from build123d import *

# Parameters (mm, degrees)
SKETCH1_W           = 15
SKETCH1_H           = 15
BOSS_EXTRUDE1_DEPTH = 2
FILLET11_R          = 5
FILLET13_R          = 2
SKETCH7_W           = 8.5
SKETCH7_H           = 7.5
BOSS_EXTRUDE5_DEPTH = 5
CUT_EXTRUDE3_DEPTH  = 5
SHELL8_T            = -0.9
FILLET15_R          = 0.45


with BuildPart() as part:
    # Sketch1 → Boss-Extrude1 (new body)
    with BuildSketch(Plane.XY):
        Rectangle(SKETCH1_W, SKETCH1_H)
    extrude(amount=BOSS_EXTRUDE1_DEPTH)

    # Fillet11
    fillet11_edges = [part.edges().sort_by_distance(p)[0] for p in [
        (7.5, -7.5, 1),
        (-7.5, -7.5, 1),
        (-7.5, 7.5, 1),
        (7.5, 7.5, 1),
    ]]
    fillet(fillet11_edges, radius=FILLET11_R)

    # Fillet13
    fillet13_edges = [part.edges().sort_by_distance(p)[0] for p in [
        (6.035533906, 6.035533906, 0),
        (0, 7.5, 0),
        (-6.035533906, 6.035533906, 0),
        (-7.5, 0, 0),
        (-6.035533906, -6.035533906, 0),
        (0, -7.5, 0),
        (6.035533906, -6.035533906, 0),
        (7.5, 0, 0),
    ]]
    fillet(fillet13_edges, radius=FILLET13_R - 0.0001)  # a hair under: the kernel refuses the full size

    # Sketch7 → Boss-Extrude5 (add)
    with BuildSketch(Plane.XY.offset(2)):
        Rectangle(SKETCH7_W, SKETCH7_H)
    extrude(amount=BOSS_EXTRUDE5_DEPTH)

    # Sketch8 → Cut-Extrude3 (cut)
    with BuildSketch(Plane.XY.offset(7)):
        Polygon((-4.25, -1.05), (-1.75, -3.75), (-4.25, -3.75), align=None)
        Polygon((4.25, -1.05), (1.75, -3.75), (4.25, -3.75), align=None)
    extrude(amount=-CUT_EXTRUDE3_DEPTH, mode=Mode.SUBTRACT)

    # Shell8
    shell8_openings = [part.faces().sort_by_distance(p)[0] for p in [
        (0, 0.3375, 7),
    ]]
    offset(amount=SHELL8_T, openings=shell8_openings, kind=Kind.INTERSECTION)

    # Fillet15
    fillet15_edges = [part.edges().sort_by_distance(p)[0] for p in [
        (0, 2.85, 7),
        (2.353387684, -1.773658698, 7),
        (-2.353387684, -1.773658698, 7),
        (0, 3.75, 7),
        (-4.25, 1.35, 7),
        (4.25, 1.35, 7),
        (0, -3.75, 7),
        (-3, -2.4, 7),
        (3, -2.4, 7),
        (-3.35, 1.076341302, 7),
        (0, -2.85, 7),
        (3.35, 1.076341302, 7),
    ]]
    fillet(fillet15_edges, radius=FILLET15_R - 0.0001)  # a hair under: the kernel refuses the full size


solid = part.part
Could you check a few things on this model? Use its own coordinates, in mm. A direction names the side the tool comes from. Coordinates: 2 decimals unless noted, no trailing zeros. Loops run counter-clockwise (first coordinate to the right, second up) from the corner with the lowest first, then second, coordinate; pieces in that order, holes last. Notation, with made-up numbers: (76.5, 13) -> (110.5, 13) arc R21 ccw to (110.5, 40) -> close; hole circle Ø11 at (-37.75, 85.25). An arc over 180 degrees is marked (long way). Answer in a Markdown table with one row per item.
(1) Thinking about a two-plate mould opening in X: for faces 1 (the face through (-2.888, -2.332, 6.865)), 2 (the face through (-2.43, -1.89, 6.87)), 3 (the face through (3, -2.4, 4.3)), which applies, released by +X, released by -X, zero draft, split by the parting line, or undercut?
Results found:
| item | result |
|---|---|
| face 1 | released by -X |
| face 2 | undercut |
| face 3 | released by +X |
(2) Imagine slicing it at A-A (z = 4). List the corners of the cut face in (x, y) for me.
Results found:
| item | result |
|---|---|
| outline | (-4.25, -1.05) -> (-1.75, -3.75) -> (1.75, -3.75) -> (4.25, -1.05) -> (4.25, 3.75) -> (-4.25, 3.75) -> close; hole (-3.35, -0.7) -> (-1.36, -2.85) -> (1.36, -2.85) -> (3.35, -0.7) -> (3.35, 2.85) -> (-3.35, 2.85) -> close |
(3) Will these pins go through, and if not, where does the flat tip stop? pin 1 Ø1 at (x, z) = (-5.5, 4) entering from -Y; pin 2 Ø2 at (x, z) = (5, 6) entering from -Y; pin 3 Ø4 at (x, z) = (-1, 4.5) entering from -Y; pin 4 Ø3 at (x, z) = (4.5, 3) entering from +Y.
Results found:
| item | result |
|---|---|
| pin 1 | passes through |
| pin 2 | stops at y = -1.32 |
| pin 3 | stops at y = -3.75 |
| pin 4 | stops at y = 7.42 |
(4) Imagine slicing it at D-D (z = 1.5). List the corners of the cut face in (x, y) for me, plus the area to 3 significant figures.
Results found:
| item | result |
|---|---|
| outline | (-7.44, -2.5) arc R4.94 ccw to (-2.5, -7.44) -> (2.5, -7.44) arc R4.94 ccw to (7.44, -2.5) -> (7.44, 2.5) arc R4.94 ccw to (2.5, 7.44) -> (-2.5, 7.44) arc R4.94 ccw to (-7.44, 2.5) -> close; hole (-3.35, -0.7) -> (-1.36, -2.85) -> (1.36, -2.85) -> (3.35, -0.7) -> (3.35, 2.85) -> (-3.35, 2.85) -> close |
| area | 166 mm^2 |
(5) For faces 4 (the face through (-3, -3, 1.1)), 5 (the face through (0.03, -6.9, 0.57)), 6 (the face through (4.25, 1, 4)), 7 (the face through (0, -3.75, 4)), 8 (the face through (3, -3, 2)), which set-ups out of +Z, -Z, +X, -X, +Y, -Y let a thin tool reach every point of the face, with its end or its side?
Results found:
| item | result |
|---|---|
| face 4 | none |
| face 5 | -Z, +X, -X, -Y |
| face 6 | +Z, +X, +Y, -Y |
| face 7 | +Z, +X, -X, -Y |
| face 8 | +Z |
(6) If I drill on probe 1 along Z at (x, y) = (3, 4); probe 2 along Y at (x, z) = (0, 4); probe 3 along Z at (x, y) = (-0.75, -2), over which ranges is the centre line in solid material (lowest first)?
Results found:
| item | result |
|---|---|
| probe 1 | z = 0 to 0.9, 1.1 to 2 |
| probe 2 | y = -3.75 to -2.85, 2.85 to 3.75 |
| probe 3 | z = 0 to 0.9 |
